Here's how the part is built. I have some questions about the finished solid (model axes, mm). A direction names the side the tool comes from. Coordinates: 2 decimals unless noted, no trailing zeros. Order: outer loops, then holes, each group sorted by start corner. A loop starts at its lowest first (then second) coordinate and runs counter-clockwise, first axis right, second up. Notation, with made-up numbers: (50, 53.25) - (79, 53.25) arc R22 cw to (79, 90.25) - close; hole circle Ø4 at (30, 82). An arc over 180 degrees is marked (long way). Use CSV: the item, a comma, the result in double quotes. Start each with the question number.
from build123d import *

# Parameters (mm, degrees)
SKETCH1_W               = 671.2712
SKETCH1_H               = 313.4106
BOSS_EXTRUDE1_DEPTH     = 15.875
SKETCH4_R               = 14.9225
CUT_EXTRUDE2_DEPTH      = 1
CUT_EXTRUDE2_DEPTH_BACK = 16.875
SKETCH5_R               = 17.4625
SKETCH5_R_2             = 2
CUT_EXTRUDE3_DEPTH      = 11.90625
SKETCH6_R               = 1.8
CUT_EXTRUDE4_DEPTH      = 2.54
SKETCH7_R               = 68
SKETCH7_R_2             = 2.54
CUT_EXTRUDE5_DEPTH      = 1
CUT_EXTRUDE5_DEPTH_BACK = 16.875
CUT_EXTRUDE6_DEPTH      = 9.525
SKETCH9_W               = 671.2712
SKETCH9_H               = 12.5
CUT_EXTRUDE7_DEPTH      = 4.35


with BuildPart() as part:
    # Sketch1 → Boss-Extrude1 (new body)
    with BuildSketch(Plane(origin=(0, 0, 0), x_dir=(1, 0, 0), z_dir=(0, 1, 0))):
        Rectangle(SKETCH1_W, SKETCH1_H)
    extrude(amount=BOSS_EXTRUDE1_DEPTH)

    # Sketch4 → Cut-Extrude2 (cut, two sides)
    with BuildSketch(Plane(origin=(0, 15.875, 0), x_dir=(1, 0, 0), z_dir=(0, 1, 0))) as cut_extrude2_sk:
        with Locations((-297.5356, -124.9553)):
            Circle(SKETCH4_R)
    extrude(amount=CUT_EXTRUDE2_DEPTH, mode=Mode.SUBTRACT)
    extrude(cut_extrude2_sk.sketch, amount=-CUT_EXTRUDE2_DEPTH_BACK, mode=Mode.SUBTRACT)

    # Sketch5 → Cut-Extrude3 (cut)
    with BuildSketch(Plane(origin=(0, 15.875, 0), x_dir=(1, 0, 0), z_dir=(0, 1, 0))):
        with Locations((0, 135.2428)):
            Circle(SKETCH5_R)
        with Locations((22.5, 125.7428)):
            Circle(SKETCH5_R_2)
        with Locations((-22.5, 125.7428)):
            Circle(SKETCH5_R_2)
        with Locations((-300, 135.2428)):
            Circle(SKETCH5_R)
        with Locations((-277.5, 125.7428)):
            Circle(SKETCH5_R_2)
        with Locations((-322.5, 125.7428)):
            Circle(SKETCH5_R_2)
        with Locations((322.5, 125.7428)):
            Circle(SKETCH5_R_2)
        with Locations((277.5, 125.7428)):
            Circle(SKETCH5_R_2)
        with Locations((300, 135.2428)):
            Circle(SKETCH5_R)
    extrude(amount=-CUT_EXTRUDE3_DEPTH, mode=Mode.SUBTRACT)

    # Sketch6 → Cut-Extrude4 (cut)
    with BuildSketch(Plane(origin=(0, 15.875, 0), x_dir=(1, 0, 0), z_dir=(0, 1, 0))):
        with Locations((78.0499912, -147.7053)):
            Circle(SKETCH6_R)
        with Locations((45.0499912, -147.7053)):
            Circle(SKETCH6_R)
        with Locations((-45.0499912, -147.7053)):
            Circle(SKETCH6_R)
        with Locations((-78.0499912, -147.7053)):
            Circle(SKETCH6_R)
    extrude(amount=-CUT_EXTRUDE4_DEPTH, mode=Mode.SUBTRACT)

    # Sketch7 → Cut-Extrude5 (cut, two sides)
    with BuildSketch(Plane(origin=(0, 15.875, 0), x_dir=(1, 0, 0), z_dir=(0, 1, 0))) as cut_extrude5_sk:
        with Locations((234.0356, 4.3053)):
            Circle(SKETCH7_R)
        with Locations((296.5356, -58.1947)):
            Circle(SKETCH7_R_2)
        with Locations((296.5356, 66.8053)):
            Circle(SKETCH7_R_2)
        with Locations((171.5356, 66.8053)):
            Circle(SKETCH7_R_2)
        with Locations((171.5356, -58.1947)):
            Circle(SKETCH7_R_2)
    extrude(amount=CUT_EXTRUDE5_DEPTH, mode=Mode.SUBTRACT)
    extrude(cut_extrude5_sk.sketch, amount=-CUT_EXTRUDE5_DEPTH_BACK, mode=Mode.SUBTRACT)

    # Sketch8 → Cut-Extrude6 (cut)
    with BuildSketch(Plane(origin=(0, 15.875, 0), x_dir=(1, 0, 0), z_dir=(0, 1, 0))):
        with BuildLine():
            Line((169.3856, -66.6947), (298.6856, -66.6947))
            ThreePointArc((298.6856, -66.6947), (303.175728061, -64.834828061), (305.0356, -60.3447))
            Line((305.0356, -60.3447), (305.0356, 68.9553))
            ThreePointArc((305.0356, 68.9553), (303.175728061, 73.445428061), (298.6856, 75.3053))
            Line((298.6856, 75.3053), (169.3856, 75.3053))
            ThreePointArc((169.3856, 75.3053), (164.895471939, 73.445428061), (163.0356, 68.9553))
            Line((163.0356, 68.9553), (163.0356, -60.3447))
            ThreePointArc((163.0356, -60.3447), (164.895471939, -64.834828061), (169.3856, -66.6947))
        make_face()
    extrude(amount=-CUT_EXTRUDE6_DEPTH, mode=Mode.SUBTRACT)

    # Sketch9 → Cut-Extrude7 (cut)
    with BuildSketch(Plane.XZ):
        with Locations((0, -91.0447)):
            Rectangle(SKETCH9_W, SKETCH9_H)
    extrude(amount=-CUT_EXTRUDE7_DEPTH, mode=Mode.SUBTRACT)


solid = part.part
Item 1: Please list where these lines run through material, in increasing order: line 1 along Z through (x, y) = (-44.5, 2); line 2 along Z through (x, y) = (-292, 10.25) (3 decimals); line 3 along Z through (x, y) = (277.5, 9.5). Write a range as from..to.
Item 2: Suppose I cut it at A-A on z = -38.5. Write out the boundary of the cut face in (x, y) (3 decimals), then the cut area to 3 significant figures.
Item 3: Suppose I cut it at C-C on x = 0. Write out the boundary of the cut face in (y, z) (3 decimals).
Item 4: Suppose I cut it at B-B on x = -300. Write out the boundary of the cut face in (y, z) (3 decimals).
Item 5: For pin 1 Ø4.5 at (x, z) = (296.54, 58.19) entering from -Y; pin 2 Ø3 at (x, z) = (22.5, -125.74) entering from +Y; pin 3 Ø1.1 at (x, z) = (45, 148) entering from +Y (3 decimals), each with a flat end and sliding along its axis, tell me the tip position at first contact or that it passes through.
Item 6: For faces 1 (the flat face through (-5, 4.35, -91)), 2 (the cylindrical face through (-299.48, 8.05, 110.16)), 3 (the cylindrical face through (286.14, 10.01, -124.62)), which set-ups out of +Z, -Z, +X, -X, +Y, -Y let a thin tool reach every point of the face, with its end or its side?
Item 7: We'd pull the mould along Z, two halves only. Please class faces 4 (the flat face through (-5, 15.875, -2)), 5 (the flat face through (-5, 8, 156.705)), 6 (the cylindrical face through (298.895, 3.219, -24.731)), 7 (the flat face through (0, 3.969, -135)): released by +Z, released by -Z, zero draft, split by the parting line, or undercut.
Here are the results:
1,line 1,"-156.71..-97.29, -84.79..156.71"
1,line 2,"-156.705..-150.765, -119.721..111.098, 138.813..156.705"
1,line 3,"-156.71..-127.74, -123.74..-75.31, 66.69..156.71"
2,outline,"(-335.636, 0) - (175.259, 0) - (175.259, 6.35) - (163.036, 6.35) - (163.036, 15.875) - (-335.636, 15.875) - close; (292.812, 0) - (335.636, 0) - (335.636, 15.875) - (305.036, 15.875) - (305.036, 6.35) - (292.812, 6.35) - close"
2,area,"8,560 mm^2"
3,outline,"(0, -156.705) - (15.875, -156.705) - (15.875, -152.705) - (3.969, -152.705) - (3.969, -117.78) - (15.875, -117.78) - (15.875, 156.705) - (0, 156.705) - (0, -84.795) - (4.35, -84.795) - (4.35, -97.295) - (0, -97.295) - close"
4,outline,"(0, -156.705) - (15.875, -156.705) - (15.875, -152.705) - (3.969, -152.705) - (3.969, -117.78) - (15.875, -117.78) - (15.875, 110.238) - (0, 110.238) - (0, -84.795) - (4.35, -84.795) - (4.35, -97.295) - (0, -97.295) - close; (0, 139.673) - (15.875, 139.673) - (15.875, 156.705) - (0, 156.705) - close"
5,pin 1,"through"
5,pin 2,"y = 3.97"
5,pin 3,"y = 13.335"
6,face 1,"+X, -X, -Y"
6,face 2,"+Y, -Y"
6,face 3,"+Y"
7,face 4,"zero draft"
7,face 5,"released by +Z"
7,face 6,"undercut"
7,face 7,"undercut"
